Geometry check sheet. Reference: the model listing, model coordinates, mm. Face numbers are marked on the shaded views. Round coordinates to 2 decimals unless told otherwise and drop trailing zeros. Order: outer loops, then holes, each group sorted by start corner. A loop starts at its lowest first (then second) coordinate and runs counter-clockwise, first axis right, second up.
(1) Release check for a two-part mould opening along X. For the marked faces 1 and 2 record: +X half, -X half, draft (parallel to the pull), parting line (faces both ways), or undercut.
(2) Sectioned sample at C-C (x = -35). Give the number of separate pieces and of enclosed holes in the cut face, plus the area to 3 significant figures.
(3) Sectioned sample at B-B (z = 8.5). Record the boundary of the cut face in (x, y).
(4) Sectioned sample at A-A (x = 4). Record the boundary of the cut face in (y, z).
(5) Material ranges on line 1 along X through (y, z) = (3.5, 32); line 2 along X through (y, z) = (-1.5, 26); line 3 along X through (y, z) = (3.75, 5), recorded low to high.
(6) Go/stop test with flat-tipped pins: pin 1 (4 mm diameter, centred on x = 5.5, z = -22.5, fed in from +Y); pin 2 (0.6 mm diameter, centred on y = 0.5, z = 3, fed in from -X); pin 3 (2 mm diameter, centred on x = 30, z = 9.5, fed in from -Y). Record where each tip stops, or that it passes through.
from build123d import *

# Parameters (mm, degrees)
SKETCH1_W            = 90
SKETCH1_H            = 70
BASE_PLATE_DEPTH     = 5
SKETCH7_R            = 2
SCREW_CUT_DEPTH      = 5
SKETCH13_W           = 48
SKETCH13_H           = 36
SCREEN_CUT_OUT_DEPTH = 10
SKETCH21_W           = 52
SKETCH21_H           = 40
SKETCH21_W_2         = 48
SKETCH21_H_2         = 36
SCREEN_MOUNT_DEPTH   = 1.25
SKETCH15_R           = 5.25
M3_NUT_OUTER_DEPTH   = 3
SKETCH18_R           = 2
SCREW_HOLE_DEPTH     = 3
M3_NUT_DEPTH         = 3
WATER_GROVES_REACH   = 85.367
SKETCH20_W           = 5
SKETCH20_H           = 2.5
FILLET1_R            = 1.5
FILLET2_R            = 1.5
FILLET3_R            = 1.5
FILLET4_R            = 1.5


with BuildPart() as part:
    # Sketch1 → Base Plate (new body)
    with BuildSketch(Plane(origin=(0, 0, 0), x_dir=(1, 0, 0), z_dir=(0, 1, 0))):
        Rectangle(SKETCH1_W, SKETCH1_H)
    extrude(amount=BASE_PLATE_DEPTH)

    # Sketch7 → Screw Cut (cut)
    with BuildSketch(Plane(origin=(0, 5, 0), x_dir=(1, 0, 0), z_dir=(0, 1, 0))):
        with Locations(Location((-36, 26, 0), (0, 0, 270))):
            Circle(SKETCH7_R)
        with Locations(Location((-36, -26, 0), (0, 0, 90))):
            Circle(SKETCH7_R)
        with Locations(Location((36, -26, 0), (0, 0, 270))):
            Circle(SKETCH7_R)
        with Locations(Location((36, 26, 0), (0, 0, 90))):
            Circle(SKETCH7_R)
    extrude(amount=-SCREW_CUT_DEPTH, mode=Mode.SUBTRACT)

    # Sketch13 → Screen Cut Out (cut)
    with BuildSketch(Plane(origin=(0, 5, 0), x_dir=(1, 0, 0), z_dir=(0, 1, 0))):
        Rectangle(SKETCH13_W, SKETCH13_H)
    extrude(amount=-SCREEN_CUT_OUT_DEPTH, mode=Mode.SUBTRACT)

    # Sketch21 → Screen Mount (cut)
    with BuildSketch(Plane.XZ):
        Rectangle(SKETCH21_W, SKETCH21_H)
        Rectangle(SKETCH21_W_2, SKETCH21_H_2, mode=Mode.SUBTRACT)
    extrude(amount=-SCREEN_MOUNT_DEPTH, mode=Mode.SUBTRACT)

    # Sketch15 → M3 Nut Outer (add)
    with BuildSketch(Plane(origin=(-42.5, 0, -25), x_dir=(1, 0, 0), z_dir=(0, -1, 0))):
        with Locations(Location((6.5, -1, 0), (0, 0, 90))):
            Circle(SKETCH15_R)
        with Locations(Location((6.5, 51, 0), (0, 0, 90))):
            Circle(SKETCH15_R)
        with Locations(Location((78.5, 51, 0), (0, 0, 90))):
            Circle(SKETCH15_R)
        with Locations(Location((78.5, -1, 0), (0, 0, 90))):
            Circle(SKETCH15_R)
    extrude(amount=M3_NUT_OUTER_DEPTH)

    # Sketch18 → Screw Hole (cut)
    with BuildSketch(Plane(origin=(0, 0, 0), x_dir=(1, 0, 0), z_dir=(0, 1, 0))):
        with Locations(Location((-36, 26, 0), (0, 0, 270))):
            Circle(SKETCH18_R)
        with Locations(Location((-36, -26, 0), (0, 0, 90))):
            Circle(SKETCH18_R)
        with Locations(Location((36, 26, 0), (0, 0, 90))):
            Circle(SKETCH18_R)
        with Locations(Location((36, -26, 0), (0, 0, 270))):
            Circle(SKETCH18_R)
    extrude(amount=-SCREW_HOLE_DEPTH, mode=Mode.SUBTRACT)

    # Sketch19 → M3 Nut (cut)
    with BuildSketch(Plane.XZ.offset(3)):
        Polygon((-36, -22.709103466), (-38.85, -24.354551733), (-38.85, -27.645448267), (-36, -29.290896534), (-33.15, -27.645448267), (-33.15, -24.354551733), align=None)
        Polygon((-33.15, 24.354551733), (-36, 22.709103466), (-38.85, 24.354551733), (-38.85, 27.645448267), (-36, 29.290896534), (-33.15, 27.645448267), align=None)
        Polygon((33.15, -24.354551733), (36, -22.709103466), (38.85, -24.354551733), (38.85, -27.645448267), (36, -29.290896534), (33.15, -27.645448267), align=None)
        Polygon((36, 22.709103466), (38.85, 24.354551733), (38.85, 27.645448267), (36, 29.290896534), (33.15, 27.645448267), (33.15, 24.354551733), align=None)
    extrude(amount=-M3_NUT_DEPTH, mode=Mode.SUBTRACT)

    # Water Groves: up to this face of the body (flat: up to its plane)
    water_groves_end = Plane(part.part.faces().sort_by_distance((0, 2.5, 35))[0])
    # Sketch20 → Water Groves (cut, up to the picked face)
    with BuildSketch(Plane(origin=(0, 0, -35), x_dir=(-1, 0, 0), z_dir=(0, 0, -1)), mode=Mode.PRIVATE) as water_groves_sk1:
        with Locations((-5.5, 3.75)):
            Rectangle(SKETCH20_W, SKETCH20_H)
    water_groves_tool1 = split(extrude(water_groves_sk1.sketch, amount=-WATER_GROVES_REACH, mode=Mode.PRIVATE), bisect_by=water_groves_end, keep=Keep.BOTH, mode=Mode.PRIVATE)
    # Sketch20 → Water Groves (cut, up to the picked face)
    with BuildSketch(Plane(origin=(0, 0, -35), x_dir=(-1, 0, 0), z_dir=(0, 0, -1)), mode=Mode.PRIVATE) as water_groves_sk2:
        with Locations((-16.5, 3.75)):
            Rectangle(SKETCH20_W, SKETCH20_H)
    water_groves_tool2 = split(extrude(water_groves_sk2.sketch, amount=-WATER_GROVES_REACH, mode=Mode.PRIVATE), bisect_by=water_groves_end, keep=Keep.BOTH, mode=Mode.PRIVATE)
    # Sketch20 → Water Groves (cut, up to the picked face)
    with BuildSketch(Plane(origin=(0, 0, -35), x_dir=(-1, 0, 0), z_dir=(0, 0, -1)), mode=Mode.PRIVATE) as water_groves_sk3:
        with Locations((16.5, 3.75)):
            Rectangle(SKETCH20_W, SKETCH20_H)
    water_groves_tool3 = split(extrude(water_groves_sk3.sketch, amount=-WATER_GROVES_REACH, mode=Mode.PRIVATE), bisect_by=water_groves_end, keep=Keep.BOTH, mode=Mode.PRIVATE)
    # Sketch20 → Water Groves (cut, up to the picked face)
    with BuildSketch(Plane(origin=(0, 0, -35), x_dir=(-1, 0, 0), z_dir=(0, 0, -1)), mode=Mode.PRIVATE) as water_groves_sk4:
        with Locations((5.5, 3.75)):
            Rectangle(SKETCH20_W, SKETCH20_H)
    water_groves_tool4 = split(extrude(water_groves_sk4.sketch, amount=-WATER_GROVES_REACH, mode=Mode.PRIVATE), bisect_by=water_groves_end, keep=Keep.BOTH, mode=Mode.PRIVATE)
    add(water_groves_tool1.solids().sort_by(Axis((5.5, 3.75, -35), (0, 0, 1)))[0], mode=Mode.SUBTRACT)
    add(water_groves_tool2.solids().sort_by(Axis((16.5, 3.75, -35), (0, 0, 1)))[0], mode=Mode.SUBTRACT)
    add(water_groves_tool3.solids().sort_by(Axis((-16.5, 3.75, -35), (0, 0, 1)))[0], mode=Mode.SUBTRACT)
    add(water_groves_tool4.solids().sort_by(Axis((-5.5, 3.75, -35), (0, 0, 1)))[0], mode=Mode.SUBTRACT)

    # Fillet1
    fillet1_edges = [part.edges().sort_by_distance(p)[0] for p in [
        (0, 0, -35),
    ]]
    fillet(fillet1_edges, radius=FILLET1_R)

    # Fillet2
    fillet2_edges = [part.edges().sort_by_distance(p)[0] for p in [
        (-45, 0, 0.75),
        (-45, 0.439339828, -34.560660172),
        (-45, 3.25, -35),
    ]]
    fillet(fillet2_edges, radius=FILLET2_R)

    # Fillet3
    fillet3_edges = [part.edges().sort_by_distance(p)[0] for p in [
        (0.75, 0, 35),
        (-44.560660172, 0.439339828, 35),
        (-45, 3.25, 35),
    ]]
    fillet(fillet3_edges, radius=FILLET3_R)

    # Fillet4
    fillet4_edges = [part.edges().sort_by_distance(p)[0] for p in [
        (45, 0.439339828, -34.560660172),
        (45, 0, 0),
        (45, 0.439339828, 34.560660172),
        (45, 3.25, -35),
        (45, 3.25, 35),
    ]]
    fillet(fillet4_edges, radius=FILLET4_R)


solid = part.part
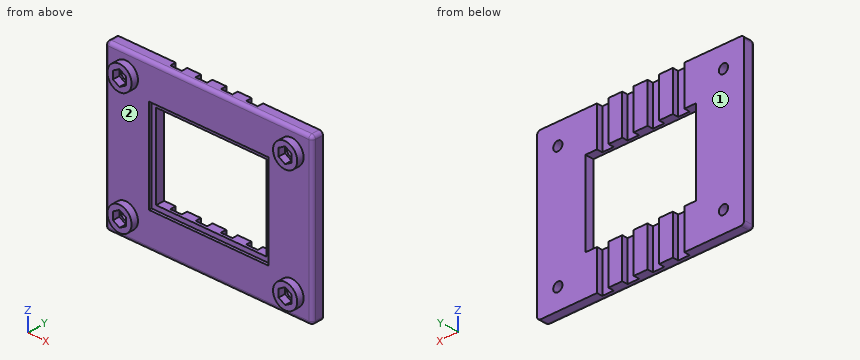
Answer below:
1. face 1: draft
1. face 2: undercut
2. separate pieces: 3
2. enclosed holes: 0
2. area: 344 mm2
3. outline: (-45, 1.5) arc R1.5 ccw to (-43.5, 0) - (-26, 0) - (-26, 1.25) - (-24, 1.25) - (-24, 5) - (-45, 5) - close; (24, 1.25) - (26, 1.25) - (26, 0) - (43.5, 0) arc R1.5 ccw to (45, 1.5) - (45, 5) - (24, 5) - close
4. outline: (0, -33.5) arc R1.5 ccw to (1.5, -35) - (2.5, -35) - (2.5, -18) - (1.25, -18) - (1.25, -20) - (0, -20) - close; (0, 20) - (1.25, 20) - (1.25, 18) - (2.5, 18) - (2.5, 35) - (1.5, 35) arc R1.5 ccw to (0, 33.5) - close
5. line 1: x = -45 to -19, -14 to -8, -3 to 3, 8 to 14, 19 to 45
5. line 2: x = -41.25 to -38.85, -33.15 to -30.75, 30.75 to 33.15, 38.85 to 41.25
5. line 3: x = -45 to -24, 24 to 45
6. pin 1: stops at y = 2.5
6. pin 2: stops at x = -44.83
6. pin 3: stops at y = 0
